Can you work these out from the drawing? Everything is in mm from the part's minimum corner. A direction names the side the tool comes from. Round coordinates to 2 decimals unless told otherwise and drop trailing zeros. Loops run counter-clockwise (first coordinate to the right, second up) from the corner with the lowest first, then second, coordinate; pieces in that order, holes last. Notation, with made-up numbers: (25, -27.75) -> (46, -27.75) arc R22 cw to (46, 9.25) -> close; hole circle Ø4 at (-18, 29). An arc over 180 degrees is marked (long way). Use CSV: the item, a comma, the result in double quotes. Start each with the question number.
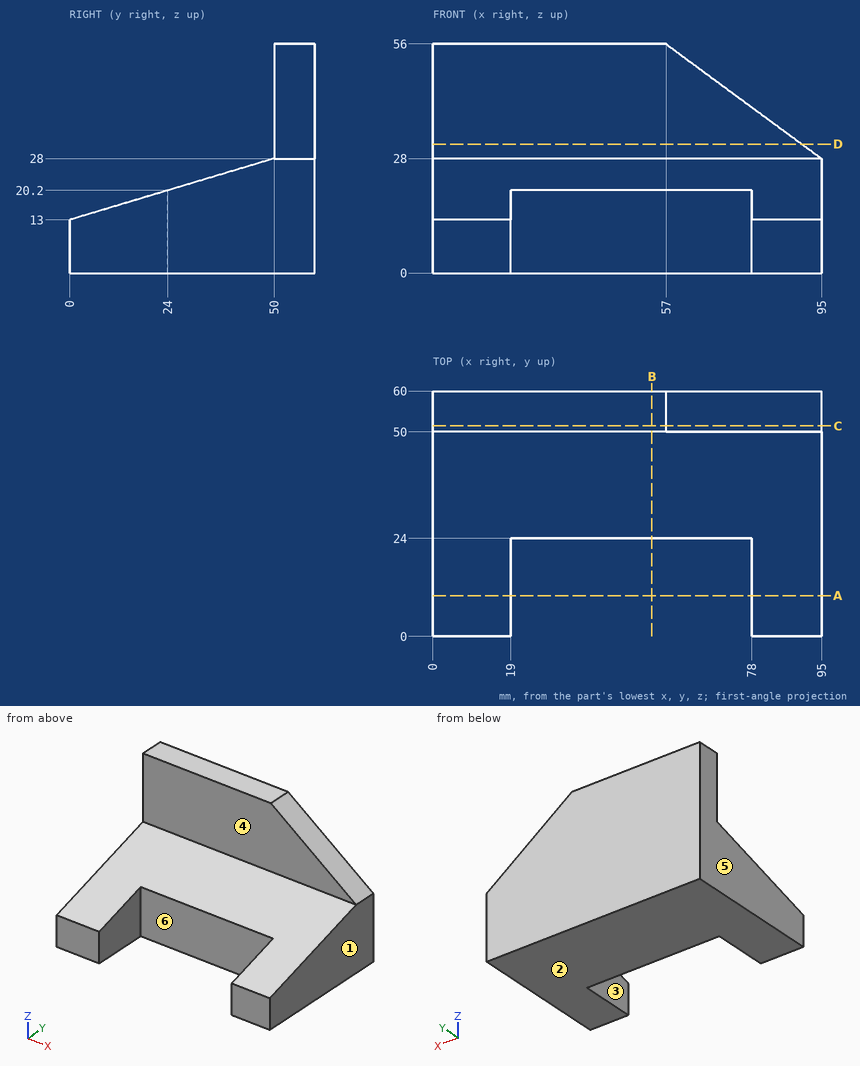
1. For the marked faces 4, 5 and 6, which set-ups out of +Z, -Z, +X, -X, +Y, -Y let a thin tool reach every point of the face, with its end or its side?
2. If I drill on L1, parallel to X at y = 21, z = 16.5; L2, parallel to Y at x = 54, z = 11; L3, parallel to Y at x = 25.5, z = 50, over which ranges is the centre line in solid material (lowest first)?
3. Suppose I cut it at A-A (y = 10). List the corners of the cut face in (x, z) for me, then the cut area to 3 significant figures.
4. Will these pins go through, and if not, where does the flat tip stop? pin 1 (2 mm diameter, centred on x = 30.5, z = 7.5, fed in from -Y); pin 2 (22.5 mm diameter, centred on x = 38.5, z = 41, fed in from -Y).
5. Suppose I cut it at C-C (y = 51.5). List the corners of the cut face in (x, z) for me.
6. We'd pull the mould along X, two halves only. Please class the marked faces 1, 2 and 3: pulls with the +X half, pulls with the -X half, needs draft (parallel to the pull), parting line crosses it, or undercut.
7. Suppose I cut it at D-D (z = 31.5). List the corners of the cut face in (x, y) for me.
8. Suppose I cut it at B-B (x = 53.5). List the corners of the cut face in (y, z) for me.
Geometry check:
1,face 4,"+Z, +X, -X, -Y"
1,face 5,"+Z, -Z, -X, +Y, -Y"
1,face 6,"+Z, -Z, -Y"
2,L1,"x = 0 to 19, 78 to 95"
2,L2,"y = 24 to 60"
2,L3,"y = 50 to 60"
3,outline,"(0, 0) -> (19, 0) -> (19, 16) -> (0, 16) -> close; (78, 0) -> (95, 0) -> (95, 16) -> (78, 16) -> close"
3,area,"576 mm²"
4,pin 1,"stops at y = 24"
4,pin 2,"stops at y = 50"
5,outline,"(0, 0) -> (95, 0) -> (95, 28) -> (57, 56) -> (0, 56) -> close"
6,face 1,"pulls with the +X half"
6,face 2,"needs draft"
6,face 3,"undercut"
7,outline,"(0, 50) -> (90.25, 50) -> (90.25, 60) -> (0, 60) -> close"
8,outline,"(24, 0) -> (60, 0) -> (60, 56) -> (50, 56) -> (50, 28) -> (24, 20.2) -> close"
